Input: part model. Units: mm. Frame: model coordinates. Face numbers are marked on the shaded views. A direction names the side the tool comes from. Give positions to 0.01 mm unless a question says otherwise; leave off trailing zeros. Loops run counter-clockwise (first coordinate to the right, second up) from the corner with the lowest first, then second, coordinate; pieces in that order, holes last. Notation, with made-up numbers: (61.25, 10.25) - (95.25, 10.25) arc R22 ccw to (95.25, 36.25) - close; hole circle Ø11 at (38.5, 58.25). An arc over 180 degrees is marked (long way). Answer as a JSON object with one key per item and string values. Group by question number.
(1) Section query B-B (x = 60.5). Return loops of the section in (y, z).
(2) Section query C-C (x = -150). Return loops of the section in (y, z), plus the area to 3 significant figures.
(3) Section query A-A (y = -10.5). Return loops of the section in (x, z).
(4) Mould query, pull axis X, two halves, no side actions, for the marked faces 1 and 2. Classes: +X half, -X half, draft (parallel to the pull), parting line (faces both ways), or undercut.
(5) Access query for the marked faces 3, 4 and 5. Directions: +Z, -Z, +X, -X, +Y, -Y. A direction counts if a zero-diameter tool reaches every point of the face in a straight line with its end or side. Return the directions, or none.
(6) Material intervals for L1, parallel to Z at x = -174.5, y = -48 (3 decimals); L2, parallel to Y at x = 188.26, z = 2; L3, parallel to X at y = -33, z = 1, sorted ascending.
(7) Pin query (flat end, axial travel): P1, Ø3, axis at x = -61, y = -57.5, coming from the -Z side; P2, Ø5, axis at x = -89.5, z = 11, coming from the +Y side; P3, Ø10, axis at x = -107.5, z = 6, coming from the -Y side; P4, Ø3.5, axis at y = -33, z = 10.5, coming from the +X side. Return the tip coordinate at first contact, or that it passes through.
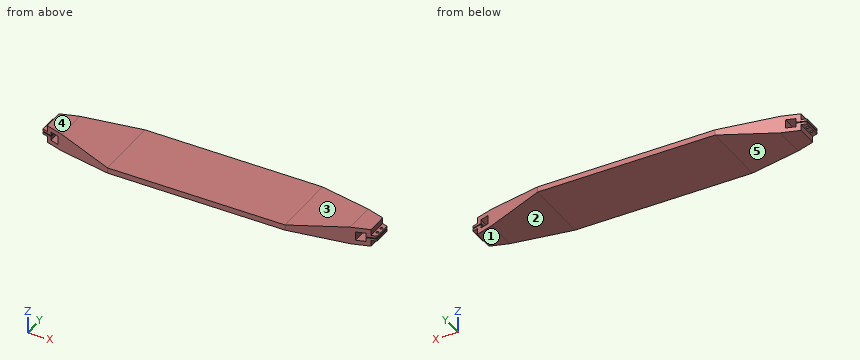
```python
from build123d import *

# Parameters (mm, degrees)
F0_W     = 6
F0_H     = 2.54
F0_W_2   = 63.5
F0_H_2   = 6.35
F0_W_3   = 101.6
F1_DEPTH = 76.2
F2_R     = 4.445
F2_R_2   = 1.5875
F3_DEPTH = 25.4
F4_R     = 1.5
F5_DEPTH = 13.121
F7_DEPTH = 20.161
F8_R     = 4.445
F8_R_2   = 1.5875
F9_DEPTH = 6.35


with BuildPart() as f1:
    # F0 (on Front) → F1 (new body)
    with BuildSketch(Plane.XZ):
        Polygon((-180.18, 3.675), (-180.18, 8.175), (-170.18, 8.175), (-170.18, -1.825), (-180.18, -1.825), (-180.18, 2.675), (-185.26, 2.675), (-185.26, 0.135), (-185.26, -6.905), (-165.1, -6.905), (-165.1, 0), (-165.1, 6.35), (-165.1, 13.255), (-185.26, 13.255), (-185.26, 6.215), (-185.26, 3.675), align=None)
        with Locations((-188.26, 4.945)):
            Rectangle(F0_W, F0_H)
        with Locations((-188.26, 1.405)):
            Rectangle(F0_W, F0_H)
        Polygon((-101.6, 6.35), (-165.1, 13.255), (-165.1, 6.35), align=None)
        with Locations((-133.35, 3.175)):
            Rectangle(F0_W_2, F0_H_2)
        with Locations((-50.8, 3.175)):
            Rectangle(F0_W_3, F0_H_2)
        Polygon((-101.6, 0), (-165.1, 0), (-165.1, -6.905), align=None)
        with Locations((50.8, 3.175)):
            Rectangle(F0_W_3, F0_H_2)
        with Locations((133.35, 3.175)):
            Rectangle(F0_W_2, F0_H_2)
        Polygon((165.1, 13.255), (101.6, 6.35), (165.1, 6.35), align=None)
        Polygon((165.1, 0), (101.6, 0), (165.1, -6.905), align=None)
        Polygon((165.1, 13.255), (165.1, 6.35), (165.1, 0), (165.1, -6.905), (185.26, -6.905), (185.26, 0.135), (185.26, 2.675), (180.18, 2.675), (180.18, -1.825), (170.18, -1.825), (170.18, 8.175), (180.18, 8.175), (180.18, 3.675), (185.26, 3.675), (185.26, 6.215), (185.26, 13.255), align=None)
        with Locations((188.26, 4.945)):
            Rectangle(F0_W, F0_H)
        with Locations((188.26, 1.405)):
            Rectangle(F0_W, F0_H)
    extrude(amount=F1_DEPTH)

    # F2 (on face) → F3 (cut)
    with BuildSketch(Plane.XY.offset(6.35)):
        with Locations((-38.1, -9.525)):
            Circle(F2_R)
        with Locations((38.1, -9.525)):
            Circle(F2_R)
        with Locations((38.1, -66.675)):
            Circle(F2_R)
        with Locations((-38.1, -66.675)):
            Circle(F2_R)
        with Locations((-22.9969, -15.1031)):
            Circle(F2_R_2)
        with Locations((22.9969, -61.0969)):
            Circle(F2_R_2)
        with Locations((22.9969, -15.1031)):
            Circle(F2_R_2)
        with Locations((-22.9969, -61.0969)):
            Circle(F2_R_2)
    extrude(amount=-F3_DEPTH, mode=Mode.SUBTRACT)

    # F4 (on face) → F5 (cut, through all)
    with BuildSketch(Plane.XY.offset(6.215)):
        with Locations((-188.26, -34.1)):
            Circle(F4_R)
        with Locations((-188.26, -42.1)):
            Circle(F4_R)
        with Locations((188.26, -42.1)):
            Circle(F4_R)
        with Locations((188.26, -34.1)):
            Circle(F4_R)
    extrude(amount=-F5_DEPTH, mode=Mode.SUBTRACT)

    # F6 (on face) → F7 (cut, through all)
    with BuildSketch(Plane.XY.offset(13.255)):
        Polygon((-165.1, -19.9012937765), (-101.6, 0), (-165.1, 0), align=None)
        Polygon((-185.26, -26.2195627928), (-165.1, -19.9012937765), (-165.1, 0), (-185.26, 0), align=None)
        Polygon((-191.26, -28.1), (-185.26, -26.2195627928), (-185.26, 0), (-191.26, 0), align=None)
        Polygon((-185.26, -76.2), (-185.26, -49.9804372072), (-191.26, -48.1), (-191.26, -76.2), align=None)
        Polygon((-165.1, -76.2), (-165.1, -56.2987062235), (-185.26, -49.9804372072), (-185.26, -76.2), align=None)
        Polygon((-101.6, -76.2), (-165.1, -56.2987062235), (-165.1, -76.2), align=None)
        Polygon((191.26, -48.1), (101.6, -76.2), (191.26, -76.2), align=None)
        Polygon((191.26, 0), (101.6, 0), (191.26, -28.1), align=None)
    extrude(amount=-F7_DEPTH, mode=Mode.SUBTRACT)

    # F8 (on face) → F9 (join, through all)
    with BuildSketch(Plane(origin=(0, 0, 0), x_dir=(1, 0, 0), z_dir=(0, 0, -1))):
        with Locations((-38.1, 66.675)):
            Circle(F8_R)
        with Locations((-38.1, 9.525)):
            Circle(F8_R)
        with Locations((-22.9969, 15.1031)):
            Circle(F8_R_2)
        with Locations((38.1, 9.525)):
            Circle(F8_R)
        with Locations((38.1, 66.675)):
            Circle(F8_R)
        with Locations((22.9969, 61.0969)):
            Circle(F8_R_2)
        with Locations((-22.9969, 61.0969)):
            Circle(F8_R_2)
        with Locations((22.9969, 15.1031)):
            Circle(F8_R_2)
    extrude(amount=-F9_DEPTH)


solid = f1.part
```
Recorded:
{
 "1": {"outline": "(-76.2, 0) - (0, 0) - (0, 6.35) - (-76.2, 6.35) - close"},
 "2": {"outline": "(-61.03, -5.26) - (-15.17, -5.26) - (-15.17, 11.61) - (-61.03, 11.61) - close", "area": "774 mm^2"},
 "3": {"outline": "(-135.1, -3.64) - (-101.6, 0) - (101.6, 0) - (135.1, -3.64) - (135.1, 9.99) - (101.6, 6.35) - (-101.6, 6.35) - (-135.1, 9.99) - close"},
 "4": {"face 1": "draft", "face 2": "undercut"},
 "5": {"face 3": "+Z, +Y, -Y", "face 4": "+Z, +X, -X, +Y, -Y", "face 5": "-Z, +Y, -Y"},
 "6": {"L1": "z = -6.905 to -1.825, 8.175 to 13.255", "L2": "y = -49.04 to -43.6, -40.6 to -35.6, -32.6 to -27.16", "L3": "x = -191.26 to -189.28, -187.24 to -180.18, -170.18 to 170.18, 180.18 to 187.24, 189.28 to 191.26"},
 "7": {"P1": "stops at z = 0", "P2": "passes through", "P3": "stops at y = -75.92", "P4": "stops at x = 185.26"}
}
